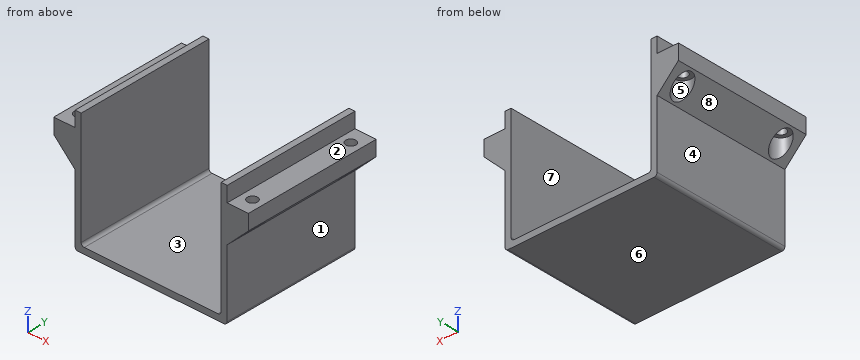
from build123d import *

# Parameters (mm, degrees)
SKETCH_1_W          = 64
SKETCH_1_H          = 40
EXTRUDE_1_DEPTH     = 45.5
CUT_EXTRUDE_1_REACH = 61.112
SKETCH_2_W          = 46
SKETCH_2_H          = 38
CUT_EXTRUDE_2_REACH = 61.112
SKETCH_3_W          = 7
SKETCH_3_H          = 30
EXTRUDE_2_DEPTH     = 45.5
CUT_EXTRUDE_3_REACH = 70.515
SKETCH_4_R          = 1.65
SKETCH_7_R          = 3
CUT_EXTRUDE_4_DEPTH = 30
SKETCH_8_W          = 7
SKETCH_8_H          = 45.5
CUT_EXTRUDE_5_DEPTH = 5
FILLET_1_R          = 1


with BuildPart() as part:
    # 草图1 → 凸台-拉伸1 (new body)
    with BuildSketch(Plane(origin=(0, 0, 0), x_dir=(1, 0, 0), z_dir=(0, 1, 0))):
        Rectangle(SKETCH_1_W, SKETCH_1_H)
    extrude(amount=EXTRUDE_1_DEPTH)

    # 草图2 → 切除-拉伸1 (cut, up to next)
    with BuildSketch(Plane(origin=(0, 45.5, 0), x_dir=(1, 0, 0), z_dir=(0, 1, 0)), mode=Mode.PRIVATE) as cut_extrude_1_sk1:
        with Locations((0, -1)):
            Rectangle(SKETCH_2_W, SKETCH_2_H)
    cut_extrude_1_tool1 = extrude(cut_extrude_1_sk1.sketch, amount=-CUT_EXTRUDE_1_REACH, mode=Mode.PRIVATE) & part.part
    add(cut_extrude_1_tool1.solids().sort_by_distance((0, 45.5, 1))[0], mode=Mode.SUBTRACT)

    # 草图3 → 切除-拉伸2 (cut, up to next)
    with BuildSketch(Plane(origin=(0, 45.5, 0), x_dir=(1, 0, 0), z_dir=(0, 1, 0)), mode=Mode.PRIVATE) as cut_extrude_2_sk1:
        with Locations((-28.5, 5)):
            Rectangle(SKETCH_3_W, SKETCH_3_H)
    cut_extrude_2_tool1 = extrude(cut_extrude_2_sk1.sketch, amount=-CUT_EXTRUDE_2_REACH, mode=Mode.PRIVATE) & part.part
    cut_extrude_2 = cut_extrude_2_tool1.solids().sort_by_distance((-28.5, 45.5, -5))[0]
    add(cut_extrude_2, mode=Mode.SUBTRACT)

    # 草图6 → 凸台-拉伸2 (add)
    with BuildSketch(Plane(origin=(0, 0, 0), x_dir=(1, 0, 0), z_dir=(0, 1, 0))):
        Polygon((-32, -10), (-25, -10), (-25, -3), align=None)
    extrude_2 = extrude(amount=EXTRUDE_2_DEPTH)

    # 切除-拉伸3: up to this plane
    cut_extrude_3_end = Plane(origin=(-25, 55.399494937, 3), z_dir=(0.7071067811865438, 0, 0.7071067811865512))
    # 草图4 → 切除-拉伸3 (cut, up to the surface)
    with BuildSketch(Plane(origin=(0, 0, 20), x_dir=(-1, 0, 0), z_dir=(0, 0, -1)), mode=Mode.PRIVATE) as cut_extrude_3_sk1:
        with Locations((28.5, 40.25)):
            Circle(SKETCH_4_R)
    cut_extrude_3_tool1 = split(extrude(cut_extrude_3_sk1.sketch, amount=CUT_EXTRUDE_3_REACH, mode=Mode.PRIVATE), bisect_by=cut_extrude_3_end, keep=Keep.BOTH, mode=Mode.PRIVATE)
    # 草图4 → 切除-拉伸3 (cut, up to the surface)
    with BuildSketch(Plane(origin=(0, 0, 20), x_dir=(-1, 0, 0), z_dir=(0, 0, -1)), mode=Mode.PRIVATE) as cut_extrude_3_sk2:
        with Locations((28.5, 5.25)):
            Circle(SKETCH_4_R)
    cut_extrude_3_tool2 = split(extrude(cut_extrude_3_sk2.sketch, amount=CUT_EXTRUDE_3_REACH, mode=Mode.PRIVATE), bisect_by=cut_extrude_3_end, keep=Keep.BOTH, mode=Mode.PRIVATE)
    cut_extrude_3 = cut_extrude_3_tool1.solids().sort_by_distance((-28.5, 40.25, 20))[0] + cut_extrude_3_tool2.solids().sort_by_distance((-28.5, 5.25, 20))[0]
    add(cut_extrude_3, mode=Mode.SUBTRACT)

    # 草图7 → 切除-拉伸4 (cut)
    with BuildSketch(Plane(origin=(0, 0, -20), x_dir=(-1, 0, 0), z_dir=(0, 0, -1))):
        with Locations((28.5, 40.25)):
            Circle(SKETCH_7_R)
        with Locations((28.5, 5.25)):
            Circle(SKETCH_7_R)
    cut_extrude_4 = extrude(amount=-CUT_EXTRUDE_4_DEPTH, mode=Mode.SUBTRACT)

    # 草图8 → 切除-拉伸5 (cut)
    with BuildSketch(Plane.XY.offset(20)):
        with Locations((-28.5, 22.75)):
            Rectangle(SKETCH_8_W, SKETCH_8_H)
    cut_extrude_5 = extrude(amount=-CUT_EXTRUDE_5_DEPTH, mode=Mode.SUBTRACT)

    # 镜向1: 切除-拉伸2, 凸台-拉伸2, 切除-拉伸3, 切除-拉伸4, 切除-拉伸5 across plane
    add(cut_extrude_2.mirror(Plane(origin=(0, 0, 0), x_dir=(0, 0, 1), z_dir=(1, 0, 0))), mode=Mode.SUBTRACT)
    add(extrude_2.mirror(Plane(origin=(0, 0, 0), x_dir=(0, 0, 1), z_dir=(1, 0, 0))))
    add(cut_extrude_3.mirror(Plane(origin=(0, 0, 0), x_dir=(0, 0, 1), z_dir=(1, 0, 0))), mode=Mode.SUBTRACT)
    add(cut_extrude_4.mirror(Plane(origin=(0, 0, 0), x_dir=(0, 0, 1), z_dir=(1, 0, 0))), mode=Mode.SUBTRACT)
    add(cut_extrude_5.mirror(Plane(origin=(0, 0, 0), x_dir=(0, 0, 1), z_dir=(1, 0, 0))), mode=Mode.SUBTRACT)

    # 圆角1
    fillet_1_edges = [part.edges().sort_by_distance(p)[0] for p in [
        (-23, 22.75, -18),
        (23, 22.75, -18),
        (-25, 22.75, -20),
        (25, 22.75, -20),
    ]]
    fillet(fillet_1_edges, radius=FILLET_1_R)


solid = part.part
Input: part model. Units: mm. Frame: model coordinates. Face numbers are marked on the shaded views. A direction names the side the tool comes from. Round coordinates to 2 decimals unless told otherwise and drop trailing zeros. Write each loop counter-clockwise with the first axis right and the second up, starting at its lowest first coordinate (ties: lowest second). Pieces come first, ordered by that corner, then holes.
1) Ray query, L1, parallel to Y at x = 28.5, z = 7.25; L2, parallel to Y at x = -28.5, z = 13.25; L3, parallel to X at y = 12, z = 0. Return the intervals inside material, ascending.
2) Cut plane D-D (y = 5.25). Count the separate pieces of the cut face and the enclosed holes in it, then the cut area to 3 significant figures.
3) Contact query for flat-ended pins moving along their axis: P1, Ø2, axis at x = -28.5, y = 22, coming from the +Z side; P2, Ø4, axis at y = 26, z = 17.5, coming from the +X side; P3, Ø6, axis at x = 10.5, y = 22.5, coming from the +Z side. Output: stop coordinate, or through.
4) Cut plane B-B (x = -28.5). Return the cut outline in (y, z).
5) Cut plane C-C (y = 24). Return the cut outline in (x, z), then the cut area to 3 significant figures.
6) Draft query along X for the marked faces 6, 7 and 8. Return one class per face: pulls with the +X half, pulls with the -X half, needs draft (parallel to the pull), parting line crosses it, or undercut.
7) Reachability of the marked faces 1, 2, 3, 4 and 5 from +Z, -Z, +X, -X, +Y, -Y: full face, straight path, thin tool, end or side. Return the list, or none.
8) Cut plane A-A (z = 17). Return the cut outline in (x, y).
Geometry says:
1. L1: y = 0 to 2.25, 8.25 to 37.25, 43.25 to 45.5
1. L2: y = 0 to 3.6, 6.9 to 38.6, 41.9 to 45.5
1. L3: x = -25 to -23, 23 to 25
2. separate pieces: 3
2. enclosed holes: 0
2. area: 296 mm2
3. P1: stops at z = 15
3. P2: stops at x = 25
3. P3: stops at z = -18
4. outline: (0, 6.5) - (2.25, 6.5) - (2.25, 10) - (3.6, 10) - (3.6, 15) - (0, 15) - close; (6.9, 10) - (8.25, 10) - (8.25, 6.5) - (37.25, 6.5) - (37.25, 10) - (38.6, 10) - (38.6, 15) - (6.9, 15) - close; (41.9, 10) - (43.25, 10) - (43.25, 6.5) - (45.5, 6.5) - (45.5, 15) - (41.9, 15) - close
5. outline: (-32, 10) - (-25, 3) - (-25, -19) arc R1 ccw to (-24, -20) - (24, -20) arc R1 ccw to (25, -19) - (25, 3) - (32, 10) - (32, 15) - (25, 15) - (25, 20) - (23, 20) - (23, -17) arc R1 cw to (22, -18) - (-22, -18) arc R1 cw to (-23, -17) - (-23, 20) - (-25, 20) - (-25, 15) - (-32, 15) - close
5. area: 371 mm2
6. face 6: needs draft
6. face 7: undercut
6. face 8: pulls with the -X half
7. face 1: -Z, +X, +Y, -Y
7. face 2: +Z, +X, +Y, -Y
7. face 3: +Z, +Y, -Y
7. face 4: -Z, -X, +Y, -Y
7. face 5: -Z
8. outline: (-25, 0) - (-23, 0) - (-23, 45.5) - (-25, 45.5) - close; (23, 0) - (25, 0) - (25, 45.5) - (23, 45.5) - close
